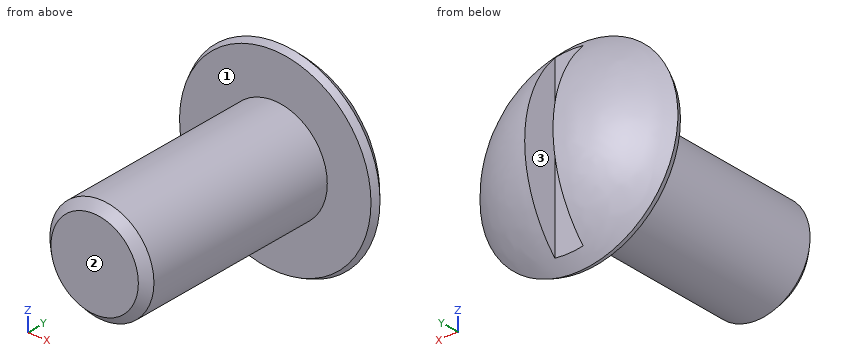
Autodesk Inventor part; units mm, degrees
ref_plane "YZ Plane" through (0, 0, 0) normal (1, 0, 0) x (0, 1, 0)
ref_plane "XZ Plane" through (0, 0, 0) normal (0, 1, 0) x (-1, 0, 0)
ref_plane "XY Plane" through (0, 0, 0) normal (0, 0, 1) x (1, 0, 0)
sketch "Sketch1" plane through (0, 0, 0) normal (0, 0, 1) x (1, 0, 0)
  line L0 (0, 7.9375) -> (0, 0)
  line L1 (0, 0) -> (1.5875, 0)
  line L2 (1.5875, 0) -> (1.5875, 6.3113)
  line L3 (1.5875, 6.3113) -> (3.175, 6.3113)
  arc A0 (3.175, 6.3113) -> (0, 7.9375) centre (0, 4.0249) ccw
  line L4 (-3.8487, 7.9375) -> (5.6755, 7.9375)
  dimension "d0" = 1.5875
  dimension "d1" = 1.5875
  dimension "d2" = 7.9375
  dimension "d10" = 3.9126
revolve "Revolution1" add sketch "Sketch1" angle 360 about axis through (0, 7.9375, 0) along (0, -1, 0)
chamfer "Chamfer1" distance 0.254 angle 45 2 edges at (-1.5875, 0, 0) (-3.175, 6.3113, 0)
sketch "Sketch2" plane through (0, 0, 0) normal (0, 0, 1) x (1, 0, 0)
  line L0 (-0.4319, 9.1026) -> (0.4319, 9.1026)
  line L1 (0.4319, 9.1026) -> (0.4319, 6.8637)
  line L2 (0.4319, 6.8637) -> (-0.4319, 6.8637)
  line L3 (-0.4319, 6.8637) -> (-0.4319, 9.1026)
  line L4 (-1.5875, 6.3113) -> (-1.5875, 0.254)
  line L5 (1.5875, 6.3113) -> (1.5875, 0.254)
  dimension "d6" = 1.1556
  dimension "d7" = 1.1556
extrude "Extrusion1" cut sketch "Sketch2" against normal mid plane 25.4
equation "\"d7\" = d6"
properties part number "screw"
Build history of the part. All positions in model axes, mm. Face numbers are marked on the shaded views. A direction names the side the tool comes from. Give positions to 0.01 mm unless a question says otherwise; leave off trailing zeros. Loops run counter-clockwise (first coordinate to the right, second up) from the corner with the lowest first, then second, coordinate; pieces in that order, holes last. Notation, with made-up numbers: (36, 27) - (74, 27) arc R5 cw to (74, 33) - close; hole circle Ø8 at (-0.75, 15). An arc over 180 degrees is marked (long way). Write item = value, one per line. Start each with the question number.
1) Drop flat-ended pins along their axis: pin 1 Ø2 at (y, z) = (2.5, 0.5) entering from +X; pin 2 Ø3 at (x, z) = (-0.5, 1) entering from -Y; pin 3 Ø1.2 at (y, z) = (7.5, 0) entering from -X; pin 4 Ø0.8 at (y, z) = (7.5, 0) entering from +X. Give the stop position or say it passes through.
2) Tool access for the marked faces 1, 2 and 3: list every direction of +Z, -Z, +X, -X, +Y, -Y with a clear straight run to the whole face (end or side of a thin tool).
3) Band-saw the part on A-A on y = 3.5. Give the cut face in (x, z) (1 decimal).
4) Probe probe 1 along Y at (x, z) = (-0.25, 0.75); probe 2 along Z at (x, y) = (0, 2.5); probe 3 along X at (y, z) = (7, 2). List the from-to ranges inside material, lowest first. Write a range as from..to.
Final values:
q1.pin_1 = 1.59
q1.pin_2 = 0
q1.pin_3 = -2.65
q1.pin_4 = 2.42
q2.face_1 = -Y
q2.face_2 = +Z, -Z, +X, -X, -Y
q2.face_3 = +Z, -Z, +Y
q3.outline = circle Ø3.2 at (0, 0)
q4.probe_1 = 0..6.86
q4.probe_2 = -1.59..1.59
q4.probe_3 = -1.57..-0.43, 0.43..1.57
